For this review, take the finished solid that the model builds, in its own axes (mm). A direction names the side the tool comes from. Coordinates: 2 decimals unless noted, no trailing zeros. Loops run counter-clockwise (first coordinate to the right, second up) from the corner with the lowest first, then second, coordinate; pieces in that order, holes last. Notation, with made-up numbers: (-37.75, -16) - (-3.75, -16) arc R22 ccw to (-3.75, -10) - close; hole circle Ø1 at (35, -26.75). An arc over 180 degrees is marked (long way). Answer as a JSON object with one key per item and string values. Group by question number.
Item 1: To check wall thickness, follow line 1 (X direction, y = -203, z = -17); line 2 (Z direction, x = 19.35, y = -590.5). State the ranges of each line that lie inside material, in increasing order.
Item 2: Mouldability with a two-part tool opening along X and no side actions: class faces 1 (the flat face through (-20, -302, 0)), 2 (the flat face through (-2, -613, -19)), 3 (the flat face through (18, -302, 0)), 4 (the flat face through (-4, -302, -18)) as released by +X, released by -X, zero draft, split by the parting line, or undercut.
Item 3: Tool access review of faces 5 (the flat face through (20, -302, 0)), 6 (the flat face through (-18, -302, 0)): name each direction out of +Z, -Z, +X, -X, +Y, -Y from which nothing blocks a thin tool from reaching the whole face with its end or side.
Item 4: We need section A-A (x = 13). Give the boundary of the cut face in (y, z), then the cut area to 3 significant figures.
Item 5: We need section B-B (y = -409). Give the boundary of the cut face in (x, z), then the cut area to 3 significant figures.
from build123d import *

# Parameters (mm, degrees)
SKETCH_W      = 40
SKETCH_H      = 40
SKETCH_W_2    = 36
SKETCH_H_2    = 36
PAD_DEPTH     = 613
SKETCH001_R   = 3.3
HOLE_DEPTH    = 40.001
SKETCH002_R   = 3.3
HOLE001_DEPTH = 40.001


with BuildPart() as part:
    # Sketch → Pad (new body)
    with BuildSketch(Plane.XZ):
        Rectangle(SKETCH_W, SKETCH_H)
        Rectangle(SKETCH_W_2, SKETCH_H_2, mode=Mode.SUBTRACT)
    extrude(amount=PAD_DEPTH)

    # Sketch001 → Hole (cut, through all)
    with BuildSketch(Plane(origin=(20, 0, 0), x_dir=(0, 0, 1), z_dir=(1, 0, 0))):
        with Locations((0, 28)):
            Circle(SKETCH001_R)
        with Locations((0, 565.5)):
            Circle(SKETCH001_R)
        with Locations((0, 590.5)):
            Circle(SKETCH001_R)
    extrude(amount=-HOLE_DEPTH, mode=Mode.SUBTRACT)

    # Sketch002 → Hole001 (cut, through all)
    with BuildSketch(Plane(origin=(0, 0, 20), x_dir=(-1, 0, 0), z_dir=(0, 0, 1))):
        with Locations((0, 15.5)):
            Circle(SKETCH002_R)
        with Locations((0, 300)):
            Circle(SKETCH002_R)
        with Locations((0, 275)):
            Circle(SKETCH002_R)
        with Locations((0, 578)):
            Circle(SKETCH002_R)
        with Locations((0, 40.5)):
            Circle(SKETCH002_R)
    extrude(amount=-HOLE001_DEPTH, mode=Mode.SUBTRACT)


solid = part.part
Check sheet entries:
{
 "1": {"line 1": "x = -20 to -18, 18 to 20", "line 2": "z = -20 to -3.3, 3.3 to 20"},
 "2": {"face 1": "released by -X", "face 2": "zero draft", "face 3": "undercut", "face 4": "undercut"},
 "3": {"face 5": "+Z, -Z, +X, +Y, -Y", "face 6": "+Y, -Y"},
 "4": {"outline": "(-613, -20) - (0, -20) - (0, -18) - (-613, -18) - close; (-613, 18) - (0, 18) - (0, 20) - (-613, 20) - close", "area": "2,450 mm2"},
 "5": {"outline": "(-20, -20) - (20, -20) - (20, 20) - (-20, 20) - close; hole (-18, -18) - (18, -18) - (18, 18) - (-18, 18) - close", "area": "304 mm2"}
}
